from build123d import *

# Parameters (mm, degrees)
F0_R     = 5
F0_R_2   = 15
F0_R_3   = 4
F1_DEPTH = 5


with BuildPart() as f1:
    # F0 (on Front) → F1 (new body)
    with BuildSketch(Plane.XZ):
        with BuildLine():
            Line((30.819411, 15.9324), (-22.541767, 24.797199))
            ThreePointArc((-22.541767, 24.797199), (-34.698621, 21.44276), (-40, 10))
            Line((-40, 10), (-40, -10))
            ThreePointArc((-40, -10), (-34.698621, -21.44276), (-22.541767, -24.797199))
            Line((-22.541767, -24.797199), (30.819411, -15.9324))
            ThreePointArc((30.819411, -15.9324), (33.814253, -14.232874), (35, -11))
            Line((35, -11), (35, 11))
            ThreePointArc((35, 11), (33.814253, 14.232874), (30.819411, 15.9324))
        make_face()
        with Locations((-25, -10)):
            Circle(F0_R, mode=Mode.SUBTRACT)
        Circle(F0_R_2, mode=Mode.SUBTRACT)
        with Locations((25, 0)):
            Circle(F0_R_3, mode=Mode.SUBTRACT)
        with Locations((-25, 10)):
            Circle(F0_R, mode=Mode.SUBTRACT)
    extrude(amount=F1_DEPTH)


solid = f1.part
The listing builds one solid part. Answer for the finished solid, in the listing's coordinates (mm). Coordinates: 2 decimals unless noted, no trailing zeros. Loops run counter-clockwise (first coordinate to the right, second up) from the corner with the lowest first, then second, coordinate; pieces in that order, holes last. Notation, with made-up numbers: M -37.75,-22 L 17.25,-22 A17 ccw 17.25,0 Z; hole C 43,56 d2. An arc over 180 degrees is marked long. Answer in a Markdown table with one row per item.
1) Find the intervals of material crossed by probe 1 along Z at (x, y) = (-25, -1.85); probe 2 along Z at (x, y) = (-24, -0.5); probe 3 along X at (y, z) = (-0.25, -12), in increasing order.
Answers below:
| item | result |
|---|---|
| probe 1 | -25 to -15, -5 to 5, 15 to 25 |
| probe 2 | -24.97 to -14.9, -5.1 to 5.1, 14.9 to 24.97 |
| probe 3 | -39.87 to -29.58, -20.42 to -9, 9 to 34.9 |
2) Find section B-B (y = -3). Determine the outline of the cut face in (x, z), then the cut area to 3 significant figures.
Answers below:
| item | result |
|---|---|
| outline | M -40,-10 A15 ccw -22.54,-24.8 L 30.82,-15.93 A5 ccw 35,-11 L 35,11 A5 ccw 30.82,15.93 L -22.54,24.8 A15 ccw -40,10 Z; hole C -25,-10 d10; hole C -25,10 d10; hole C 0,0 d30; hole C 25,0 d8 |
| area | 2,160 mm^2 |
3) Find section A-A (z = 0). Determine the outline of the cut face in (x, y).
Answers below:
| item | result |
|---|---|
| outline | M -40,-5 L -15,-5 L -15,0 L -40,0 Z; M 15,-5 L 21,-5 L 21,0 L 15,0 Z; M 29,-5 L 35,-5 L 35,0 L 29,0 Z |
4) Find section D-D (x = 25). Determine the outline of the cut face in (y, z), then the cut area to 3 significant figures.
Answers below:
| item | result |
|---|---|
| outline | M -5,-16.9 L 0,-16.9 L 0,-4 L -5,-4 Z; M -5,4 L 0,4 L 0,16.9 L -5,16.9 Z |
| area | 129 mm^2 |
5) Find section C-C (x = 1). Determine the outline of the cut face in (y, z), then the cut area to 3 significant figures.
Answers below:
| item | result |
|---|---|
| outline | M -5,-20.89 L 0,-20.89 L 0,-14.97 L -5,-14.97 Z; M -5,14.97 L 0,14.97 L 0,20.89 L -5,20.89 Z |
| area | 59.2 mm^2 |
6) Determine the mould class of faces 1 (the cylindrical face through (-30, -2, 10)), 2 (the flat face through (3.765, -2.465, -20.427)), 3 (the flat face through (4.512, -2.465, 20.303)) for opening direction Z: released by +Z, released by -Z, zero draft, split by the parting line, or undercut.
Answers below:
| item | result |
|---|---|
| face 1 | undercut |
| face 2 | released by -Z |
| face 3 | released by +Z |
7) Given pin 1 (1.5 mm diameter, centred on x = 12.5, y = -1, fed in from +Z); pin 2 (8 mm diameter, centred on x = 2.5, z = -9.5, fed in from +Y); pin 3 (2 mm diameter, centred on x = -28.5, y = -2, fed in from +Z), each flat-ended and moving along its own axis, determine where each tip first touches the part or whether it passes through.
Answers below:
| item | result |
|---|---|
| pin 1 | z = 19.1 |
| pin 2 | through |
| pin 3 | z = 24.79 |
